Part model, mm, in its own coordinate system. Face numbers are marked on the shaded views. A direction names the side the tool comes from. Coordinates: 2 decimals unless noted, no trailing zeros. Order: outer loops, then holes, each group sorted by start corner. A loop starts at its lowest first (then second) coordinate and runs counter-clockwise, first axis right, second up.
1) Cut at C-C (y = -28). List the corners of the cut face in (x, z), and give its area (3 significant figures).
2) Mould opens along Y. For the marked faces 1, 2 and 3 say: +Y half, -Y half, draft (parallel to the pull), parting line (faces both ways), or undercut.
3) Wall check: L1, parallel to Y at x = 19.5, z = 6; L2, parallel to X at y = -49, z = 1.75; L3, parallel to X at y = -21.5, z = 4.25 (3 decimals). Give the ranges that are in metal, low to high.
4) Cut at A-A (x = 2). List the corners of the cut face in (y, z).
5) Cut at D-D (z = 1.25). Give the number of separate pieces and of enclosed holes in the cut face, and give its area (3 significant figures).
6) Tool access for the marked faces 4 and 5: list every direction of +Z, -Z, +X, -X, +Y, -Y with a clear straight run to the whole face (end or side of a thin tool).
7) Pin check, flat tips, straight feed: pin 1 Ø3.5 at (y, z) = (-44, 4) entering from +X; pin 2 Ø3 at (y, z) = (-5.5, 2.5) entering from +X; pin 3 Ø2.5 at (y, z) = (-4, 2) entering from -X. Stop position of each tip, or through.
8) Cut at B-B (y = -44). List the corners of the cut face in (x, z).
```python
from build123d import *

# Parameters (mm, degrees)
BOSS_EXTRUDE1_DEPTH     = 6.5532
CUT_EXTRUDE1_DEPTH      = 94.204461666
CUT_EXTRUDE2_DEPTH      = 94.204461666
CUT_EXTRUDE3_DEPTH      = 94.204461666
CUT_EXTRUDE4_DEPTH      = 94.204461666
F_1_4_CLEARANCE_HOLE1_D = 6.604
HOLE1_D                 = 4.953
HOLE2_D                 = 22.1996
HOLE2_CBORE_D           = 25.019
HOLE2_CBORE_DEPTH       = 1.5875
FILLET1_R               = 3.302


with BuildPart() as part:
    # Sketch1 → Boss-Extrude1 (new body)
    with BuildSketch(Plane.XY.offset(6.5532)):
        with BuildLine():
            Line((24.389857327, -74.032249917), (50.14347414, -0.124279011))
            Line((50.14347414, -0.124279011), (50.14347414, 9.400720989))
            Line((50.14347414, 9.400720989), (-13.35652586, 9.400720989))
            Line((-13.35652586, 9.400720989), (-13.35652586, -0.124279011))
            Line((-13.35652586, -0.124279011), (12.397090952, -74.032249917))
            ThreePointArc((12.397090952, -74.032249917), (18.39347414, -78.292779011), (24.389857327, -74.032249917))
        make_face()
    extrude(amount=-BOSS_EXTRUDE1_DEPTH)

    # Sketch2 → Cut-Extrude1 (cut, through all)
    with BuildSketch(Plane.XY.offset(6.5532)):
        with BuildLine():
            Line((20.61597414, -35.794091329), (20.61597414, -51.420905267))
            ThreePointArc((20.61597414, -51.420905267), (23.377652776, -54.67839768), (27.043143627, -52.486982035))
            Line((27.043143627, -52.486982035), (32.590050314, -36.226404888))
            ThreePointArc((32.590050314, -36.226404888), (31.312054869, -32.423331215), (27.307035446, -32.660946735))
            ThreePointArc((27.307035446, -32.660946735), (24.177686628, -34.689191283), (20.61597414, -35.794091329))
        make_face()
    extrude(amount=-CUT_EXTRUDE1_DEPTH, mode=Mode.SUBTRACT)

    # Sketch3 → Cut-Extrude2 (cut, through all)
    with BuildSketch(Plane.XY.offset(6.5532)):
        with BuildLine():
            Line((16.17097414, -51.420905267), (16.17097414, -35.794091329))
            ThreePointArc((16.17097414, -35.794091329), (12.609261651, -34.689191283), (9.479912834, -32.660946735))
            ThreePointArc((9.479912834, -32.660946735), (5.47489341, -32.423331215), (4.196897965, -36.226404888))
            Line((4.196897965, -36.226404888), (9.743804652, -52.486982035))
            ThreePointArc((9.743804652, -52.486982035), (13.409295504, -54.67839768), (16.17097414, -51.420905267))
        make_face()
    extrude(amount=-CUT_EXTRUDE2_DEPTH, mode=Mode.SUBTRACT)

    # Sketch4 → Cut-Extrude3 (cut, through all)
    with BuildSketch(Plane.XY.offset(6.5532)):
        with BuildLine():
            Line((38.119000553, -20.018466488), (43.427416008, -4.457018658))
            ThreePointArc((43.427416008, -4.457018658), (42.991263585, -1.493779513), (40.327528698, -0.124279011))
            Line((40.327528698, -0.124279011), (20.61597414, -0.124279011))
            Line((20.61597414, -0.124279011), (20.61597414, -8.879066693))
            ThreePointArc((20.61597414, -8.879066693), (27.856065704, -12.512959264), (31.758379191, -19.611976838))
            ThreePointArc((31.758379191, -19.611976838), (34.783239019, -22.2476674), (38.119000553, -20.018466488))
        make_face()
    extrude(amount=-CUT_EXTRUDE3_DEPTH, mode=Mode.SUBTRACT)

    # Sketch5 → Cut-Extrude4 (cut, through all)
    with BuildSketch(Plane(origin=(0, 0, 0), x_dir=(-1, 0, 0), z_dir=(0, 0, -1))):
        with BuildLine():
            Line((1.332052274, -20.018466488), (6.640467729, -4.457018658))
            ThreePointArc((6.640467729, -4.457018658), (6.204315306, -1.493779513), (3.540580419, -0.124279011))
            Line((3.540580419, -0.124279011), (-16.17097414, -0.124279011))
            Line((-16.17097414, -0.124279011), (-16.17097414, -8.879066693))
            ThreePointArc((-16.17097414, -8.879066693), (-8.930882576, -12.512959264), (-5.028569088, -19.611976838))
            ThreePointArc((-5.028569088, -19.611976838), (-2.00370926, -22.2476674), (1.332052274, -20.018466488))
        make_face()
    extrude(amount=-CUT_EXTRUDE4_DEPTH, mode=Mode.SUBTRACT)

    # 1/4 Clearance Hole1 (through all)
    with Locations(Plane(origin=(0, 0, 0), x_dir=(-1, 0, 0), z_dir=(0, 0, -1))):
        with Locations((-18.39347414, -71.942579011)):
            Hole(F_1_4_CLEARANCE_HOLE1_D / 2)

    # Hole1 (through all)
    with Locations(Plane.XY.offset(6.5532)):
        with Locations((9.92765366, 4.638220989), (26.85929426, 4.638220989), (-7.00652586, 4.638220989), (43.79347426, 4.638220989)):
            Hole(HOLE1_D / 2)

    # Hole2 (through all)
    with Locations(Plane.XY.offset(6.5532)):
        with Locations((18.39347414, -22.336579011)):
            CounterBoreHole(HOLE2_D / 2, HOLE2_CBORE_D / 2, HOLE2_CBORE_DEPTH)

    # Fillet1
    fillet1_edges = [part.edges().sort_by_distance(p)[0] for p in [
        (20.61597414, -35.794091329, 3.2766),
        (16.17097414, -35.794091329, 3.2766),
        (20.61597414, -8.879066693, 3.2766),
        (20.61597414, -0.124279011, 3.2766),
        (16.17097414, -8.879066693, 3.2766),
        (16.17097414, -0.124279011, 3.2766),
    ]]
    fillet(fillet1_edges, radius=FILLET1_R)


solid = part.part
```
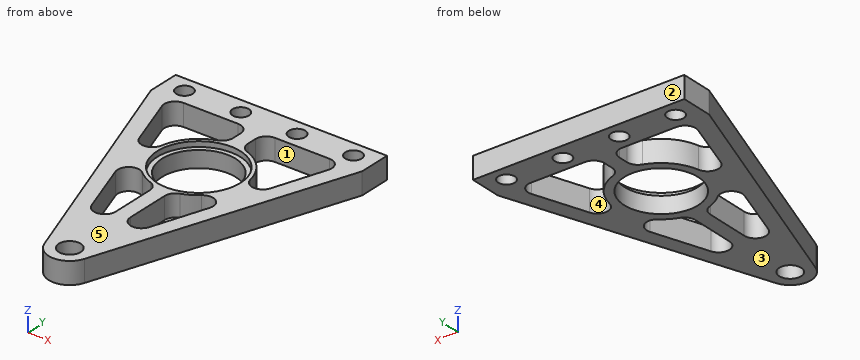
Geometry check:
1. outline: (-3.64, 0) - (8.85, 0) - (8.85, 4.97) - (7.24, 4.97) - (7.24, 6.55) - (-3.64, 6.55) - close; (27.94, 0) - (40.43, 0) - (40.43, 6.55) - (29.55, 6.55) - (29.55, 4.97) - (27.94, 4.97) - close
1. area: 159 mm2
2. face 1: undercut
2. face 2: +Y half
2. face 3: draft
3. L1: y = -78.2 to -75.05, -68.83 to -34.8, -9.88 to 9.4
3. L2: x = 3.67 to 8.55, 16.17 to 20.62, 28.23 to 33.11
3. L3: x = -5.908 to -0.308, 3.894 to 7.325, 29.462 to 32.893, 37.095 to 42.695
4. outline: (-44.19, 0) - (-22.25, 0) - (-22.25, 6.55) - (-44.19, 6.55) - close; (-0.12, 0) - (9.4, 0) - (9.4, 6.55) - (-0.12, 6.55) - close
5. separate pieces: 1
5. enclosed holes: 10
5. area: 1,900 mm2
6. face 4: +Z, -Z
6. face 5: +Z, +X, -X, +Y, -Y
7. pin 1: stops at x = 35.46
7. pin 2: stops at x = 48.79
7. pin 3: stops at x = -12.44
8. outline: (1.93, 0) - (6.85, 0) - (6.85, 6.55) - (1.93, 6.55) - close; (16.17, 0) - (20.62, 0) - (20.62, 6.55) - (16.17, 6.55) - close; (29.94, 0) - (34.85, 0) - (34.85, 6.55) - (29.94, 6.55) - close
